Here's how the part is built. I have some questions about the finished solid (model axes, mm). Face numbers are marked on the shaded views. A direction names the side the tool comes from. Coordinates: 2 decimals unless noted, no trailing zeros. Write each loop counter-clockwise with the first axis right and the second up, starting at its lowest first coordinate (ties: lowest second). Pieces come first, ordered by that corner, then holes.
Item 1: For the marked faces 4 and 5, which set-ups out of +Z, -Z, +X, -X, +Y, -Y let a thin tool reach every point of the face, with its end or its side?
Item 2: If I drill on line 1 (Z direction, x = -1, y = 10); line 2 (Z direction, x = -7, y = 13.2); line 3 (Z direction, x = -1, y = 19.5), over which ranges is the centre line in solid material (lowest first)?
Item 3: If we section it at A-A (z = 0): Please give me the cut outline in (x, y), then the cut area to 4 significant figures.
Item 4: If we section it at B-B (x = 0): Please give me the cut outline in (y, z).
Item 5: If we section it at C-C (y = 2.5): Please give me the cut outline in (x, z), then the cut area to 3 significant figures.
Item 6: We'd pull the mould along X, two halves only. Please class the marked faces 1, 2 and 3: +X half, -X half, draft (parallel to the pull), parting line (faces both ways), or undercut.
Item 7: I'm going to push flat-ended pins straight in: pin 1 Ø20 at (x, z) = (20.5, -2) entering from +Y; pin 2 Ø10 at (x, y) = (-24, 16.5) entering from -Z; pin 3 Ø4 at (y, z) = (25.5, 3) entering from -X. Where does each tip first touch, or does it pass through?
Item 8: If we section it at D-D (y = 27): Please give me the cut outline in (x, z) (3 decimals), then the cut area to 3 significant figures.
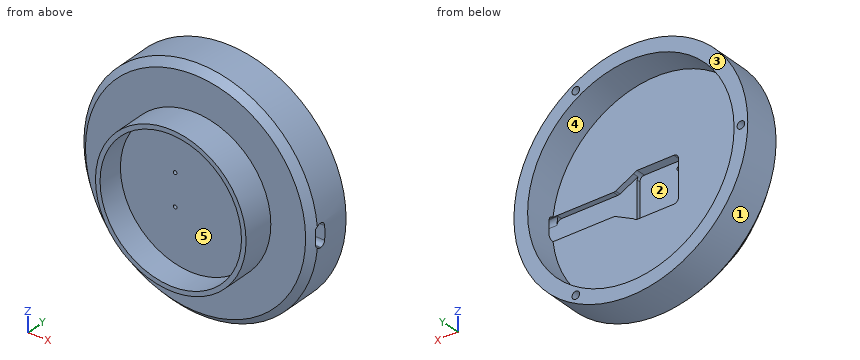
from build123d import *

# Parameters (mm, degrees)
TROU_POUR_TARAUDAGE_POUR_TROU_TARAUD_M4_D     = 3.3
TROU_POUR_TARAUDAGE_POUR_TROU_TARAUD_M4_DEPTH = 10
CHANFREIN1_SIZE                               = 3
ENL_V_MAT_EXTRU_1_DEPTH                       = 4
ENL_V_START                                   = -2.5
ENL_V_MAT_EXTRU_2_DEPTH                       = 2.5
TROU_POUR_TARAUDAGE_POUR_TROU_TARAUD_M2_D     = 1.6
ENL_V_MAT_EXTRU_3_REACH                       = 121.255


with BuildPart() as part:
    # Esquisse1 → Révolution1 (revolve)
    with BuildSketch(Plane.XY):
        Polygon((0, 11.5), (31, 11.5), (31, 0), (33, 0), (33, 14), (51.25, 14), (51.25, 33), (45.25, 33), (45.25, 19), (0, 19), align=None)
    revolve(axis=Axis((0, 0, 0), (0, 1, 0)))

    # Trou pour taraudage pour trou taraudé M41
    with Locations(Plane(origin=(0, 33, 0), x_dir=(1, 0, 0), z_dir=(0, 1, 0))):
        with Locations((-48.25, 0), (24.125, 41.785725733), (24.125, -41.785725733)):
            Hole(TROU_POUR_TARAUDAGE_POUR_TROU_TARAUD_M4_D / 2, depth=TROU_POUR_TARAUDAGE_POUR_TROU_TARAUD_M4_DEPTH)

    # Chanfrein1
    chanfrein1_edges = [part.edges().sort_by_distance(p)[0] for p in [
        (-51.25, 14, 0),
    ]]
    chamfer(chanfrein1_edges, length=CHANFREIN1_SIZE)

    # Esquisse4 → Enlèv. mat.-Extru.1 (cut)
    with BuildSketch(Plane(origin=(0, 19, 0), x_dir=(1, 0, 0), z_dir=(0, 1, 0))):
        with BuildLine():
            Line((-8, 10), (8, 10))
            ThreePointArc((8, 10), (9.414213562, 9.414213562), (10, 8))
            Line((10, 8), (10, -8))
            ThreePointArc((10, -8), (9.414213562, -9.414213562), (8, -10))
            Line((8, -10), (-8, -10))
            ThreePointArc((-8, -10), (-9.414213562, -9.414213562), (-10, -8))
            Line((-10, -8), (-10, 8))
            ThreePointArc((-10, 8), (-9.414213562, 9.414213562), (-8, 10))
        make_face()
    extrude(amount=-ENL_V_MAT_EXTRU_1_DEPTH, mode=Mode.SUBTRACT)

    # Esquisse5 → Enlèv. mat.-Extru.2 (cut)
    with BuildSketch(Plane(origin=(0, 19, 0), x_dir=(1, 0, 0), z_dir=(0, 1, 0)).offset(ENL_V_START)):
        with BuildLine():
            Line((8, -10), (17.577708764, -5.211145618))
            ThreePointArc((17.577708764, -5.211145618), (18.012630114, -5.053502021), (18.472135955, -5))
            Line((18.472135955, -5), (43.145828304, -5))
            ThreePointArc((43.145828304, -5), (44.510112613, -4.462439169), (45.141011115, -3.138728324))
            ThreePointArc((45.141011115, -3.138728324), (45.25, 0), (45.141011115, 3.138728324))
            ThreePointArc((45.141011115, 3.138728324), (44.510112613, 4.462439169), (43.145828304, 5))
            Line((43.145828304, 5), (18.472135955, 5))
            ThreePointArc((18.472135955, 5), (18.012630114, 5.053502021), (17.577708764, 5.211145618))
            Line((17.577708764, 5.211145618), (8, 10))
            Line((8, 10), (8, -10))
        make_face()
    extrude(amount=ENL_V_MAT_EXTRU_2_DEPTH, mode=Mode.SUBTRACT)

    # Trou pour taraudage pour trou taraudé M21 (through all)
    with Locations(Plane(origin=(0, 15, 0), x_dir=(1, 0, 0), z_dir=(0, 1, 0))):
        with Locations((-7, 7), (-7, -7)):
            Hole(TROU_POUR_TARAUDAGE_POUR_TROU_TARAUD_M2_D / 2)

    # Esquisse8 → Enlèv. mat.-Extru.3 (cut, up to next)
    with BuildSketch(Plane(origin=(51.25, 0, 0), x_dir=(0, 0, -1), z_dir=(1, 0, 0)), mode=Mode.PRIVATE) as enl_v_mat_extru_3_sk1:
        with BuildLine():
            Line((-3, 21), (3, 21))
            ThreePointArc((3, 21), (4.414213562, 20.414213562), (5, 19))
            Line((5, 19), (5, 18.5))
            ThreePointArc((5, 18.5), (4.414213562, 17.085786438), (3, 16.5))
            Line((3, 16.5), (-3, 16.5))
            ThreePointArc((-3, 16.5), (-4.414213562, 17.085786438), (-5, 18.5))
            Line((-5, 18.5), (-5, 19))
            ThreePointArc((-5, 19), (-4.414213562, 20.414213562), (-3, 21))
        make_face()
    enl_v_mat_extru_3_tool1 = extrude(enl_v_mat_extru_3_sk1.sketch, amount=-ENL_V_MAT_EXTRU_3_REACH, mode=Mode.PRIVATE) & part.part
    add(enl_v_mat_extru_3_tool1.solids().sort_by_distance((51.25, 18.75, 0))[0], mode=Mode.SUBTRACT)


solid = part.part
Answer list:
1. face 4: +Y
1. face 5: -Y
2. line 1: z = -32.98 to -30.98, 30.98 to 32.98
2. line 2: z = -32.25 to -7.8, -6.2 to 6.2, 7.8 to 32.25
2. line 3: z = -51.24 to -45.24, 45.24 to 51.24
3. outline: (-51.25, 17) - (-48.25, 14) - (-33, 14) - (-33, 0) - (-31, 0) - (-31, 11.5) - (31, 11.5) - (31, 0) - (33, 0) - (33, 14) - (48.25, 14) - (50.75, 16.5) - (10, 16.5) - (10, 15) - (-10, 15) - (-10, 19) - (-45.25, 19) - (-45.25, 33) - (-46.6, 33) - (-46.6, 23) - (-49.9, 23) - (-49.9, 33) - (-51.25, 33) - close; (45.25, 21) - (51.25, 21) - (51.25, 33) - (45.25, 33) - close
3. area: 654.5 mm2
4. outline: (0, -33) - (14, -33) - (14, -48.25) - (17, -51.25) - (33, -51.25) - (33, -45.25) - (19, -45.25) - (19, -10) - (15, -10) - (15, 10) - (19, 10) - (19, 45.25) - (33, 45.25) - (33, 51.25) - (17, 51.25) - (14, 48.25) - (14, 33) - (0, 33) - (0, 31) - (11.5, 31) - (11.5, -31) - (0, -31) - close
5. outline: circle Ø66 at (0, 0); hole circle Ø62 at (0, 0)
5. area: 402 mm2
6. face 1: parting line
6. face 2: undercut
6. face 3: draft
7. pin 1: stops at y = 19
7. pin 2: stops at z = -47.59
7. pin 3: stops at x = -51.24
8. outline: circle Ø102.5 at (0, 0); hole circle Ø3.3 at (-48.25, 0); hole circle Ø90.5 at (0, 0); hole circle Ø3.3 at (24.125, -41.786); hole circle Ø3.3 at (24.125, 41.786)
8. area: 1,790 mm2
